from build123d import *

# Parameters (mm, degrees)
F1_DEPTH = 25.4
F2_SIZE  = 25.39999
F4_DEPTH = 99.314
F5_SIZE2 = 99.2610316746
F5_SIZE  = 40.10406


# Not quite as in the source:
# - a fillet or chamfer is up to 0.001 mm smaller than in the source, because OpenCascade refuses the exact size


with BuildPart() as f1:
    # F0 (on Top) → F1 (new body)
    with BuildSketch(Plane.XY):
        Polygon((40.3215661799, -64.3411021127), (74.0076824868, -16.984376739), (64.3411021127, 40.3215661799), (16.984376739, 74.0076824868), (-40.3215661799, 64.3411021127), (-74.0076824868, 16.984376739), (-64.3411021127, -40.3215661799), (-16.984376739, -74.0076824868), align=None)
    extrude(amount=F1_DEPTH)

    # F2 (size 25.4 in the source; OpenCascade refuses exactly that, so slightly less here)
    f2_edges = [f1.edges().sort_by_distance(p)[0] for p in [
        (11.668595, -69.174392, 25.4),
        (57.164624, -40.662739, 25.4),
        (69.174392, 11.668595, 25.4),
        (40.662739, 57.164624, 25.4),
        (-11.668595, 69.174392, 25.4),
        (-69.174392, -11.668595, 25.4),
        (-40.662739, -57.164624, 25.4),
        (-57.164624, 40.662739, 25.4),
    ]]
    chamfer(f2_edges, length=F2_SIZE)

    # F3 (on face) → F4 (join)
    with BuildSketch(Plane.XY.offset(25.4)):
        Polygon((-18.6424832791, 25.9398680102), (0, -26.7094988376), (25.9398680102, 23.150825873), align=None)
    extrude(amount=F4_DEPTH)

    # F5
    f5_edges = [f1.edges().sort_by_distance(p)[0] for p in [
        (-9.321242, -0.384815, 124.714),
    ]]
    f5_side = f1.faces().sort_by_distance((2.432462, 7.460398, 124.714))[0]
    chamfer(f5_edges, length=F5_SIZE, length2=F5_SIZE2, reference=f5_side)


solid = f1.part
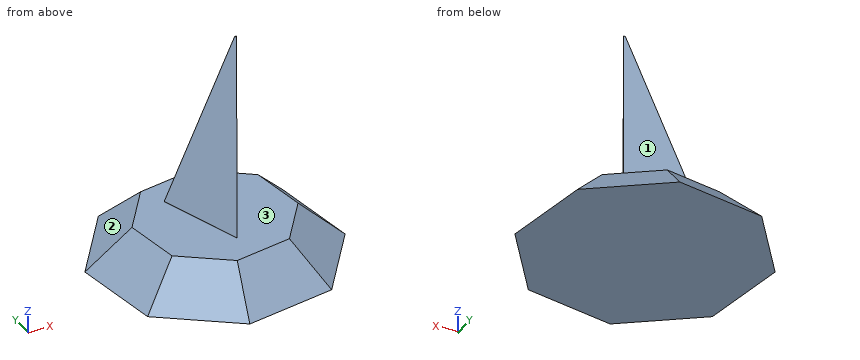
Read the model definition and answer for the solid it produces. Units are mm, in the model's axes. Face numbers are marked on the shaded views. A direction names the side the tool comes from. Give positions to 0.01 mm unless a question says otherwise; leave off trailing zeros. Loops run counter-clockwise (first coordinate to the right, second up) from the corner with the lowest first, then second, coordinate; pieces in that order, holes last. Notation, with made-up numbers: (49.25, 22) - (53.25, 22) arc R22 cw to (53.25, 57) - close; hole circle Ø1 at (37, -25). An arc over 180 degrees is marked (long way). Answer as CSV lines item,"result". Start each with the question number.
1) Which of the six approach directions +Z, -Z, +X, -X, +Y, -Y give full straight-line access (tool end or side, diameter ignored) to the marked faces 1, 2 and 3?
2) Find section C-C (z = 19). Write down the section's boundary in (x, y), then the cut area to 3 significant figures.
3) Each of these flat-tipped pins is pushed along its axis until it touches: pin 1 Ø1.5 at (x, y) = (17.5, -13) entering from +Z; pin 2 Ø1.5 at (x, z) = (-2.5, 31) entering from +Y; pin 3 Ø8 at (y, z) = (24, 35.5) entering from -X. Where does it stop, or does it pass through?
4) Straight lines are drawn through the part: L1, parallel to Z at x = -18, y = -37; L2, parallel to Y at x = 18.5, z = 76.5; L3, parallel to X at y = 8, z = 83. For each, find the intervals that lie inside material, in ascending order. Write a range as from..to.
Findings below:
1,face 1,"+Z, +X, +Y"
1,face 2,"+Z, -X, +Y"
1,face 3,"+Z"
2,outline,"(-53.96, 12.38) - (-46.91, -29.4) - (-12.38, -53.96) - (29.4, -46.91) - (53.96, -12.38) - (46.91, 29.4) - (12.38, 53.96) - (-29.4, 46.91) - close"
2,area,"8,670 mm^2"
3,pin 1,"z = 25.4"
3,pin 2,"y = 24.98"
3,pin 3,"x = -15.81"
4,L1,"0..25.4"
4,L2,"8.85..23.62"
4,L3,"12.37..18.06"
